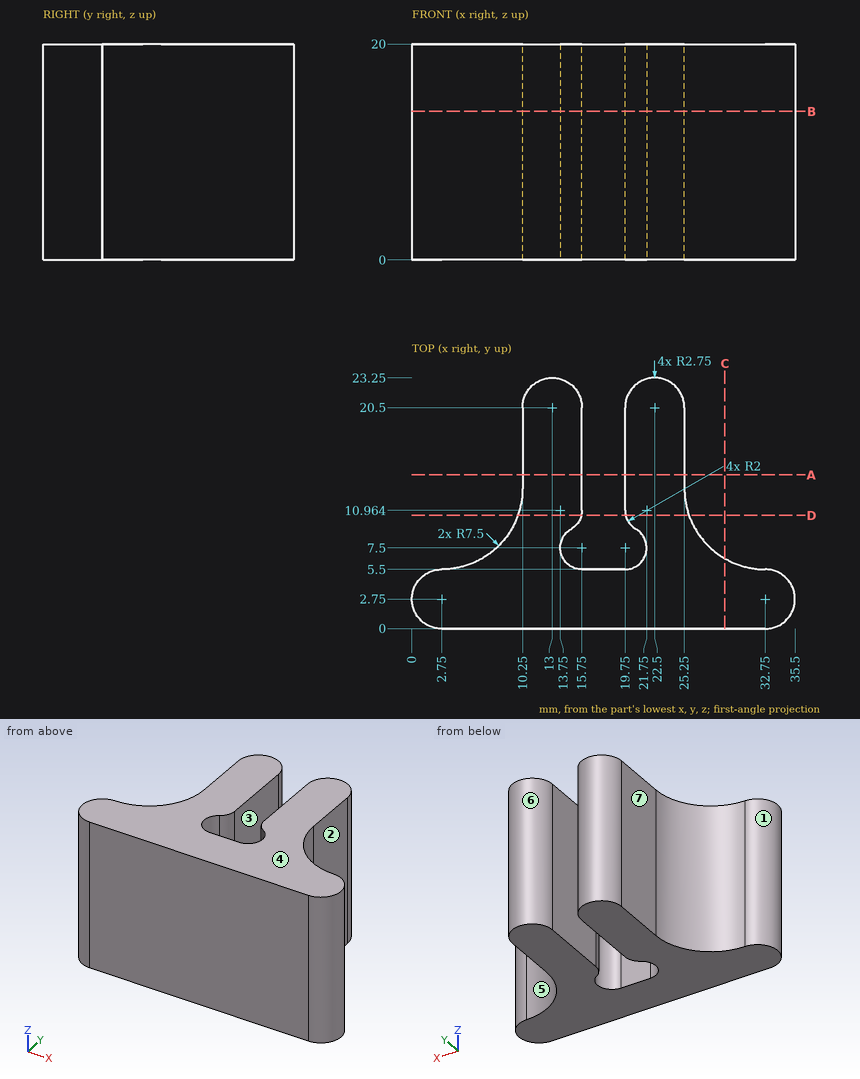
For this review, use the dimensioned drawing (mm, ordinates from the lowest corner) and the shaded views. A direction names the side the tool comes from. Give positions to 0.01 mm unless a question says otherwise; leave off trailing zeros. Order: outer loops, then holes, each group sorted by start corner. A loop starts at its lowest first (then second) coordinate and runs counter-clockwise, first axis right, second up. Notation, with made-up numbers: M 33,-40 L 85,-40 A12 ccw 85,-17 Z; hole C -22,62.5 d10. An arc over 180 degrees is marked long. Use one line per item in the form item = value. Start each with the question number.
Item 1: Insertion check: pin 1 Ø3 at (x, z) = (18, 15) entering from +Y; pin 2 Ø1 at (y, z) = (17, 8) entering from -X; pin 3 Ø1.5 at (y, z) = (15.5, 3.5) entering from +X. Each pin has a flat end and moves straight along its axis. Give the tip position at first contact, or say it passes through.
Item 2: We need section C-C on x = 29. Give the boundary of the cut face in (y, z) (3 decimals).
Item 3: For the marked faces 1, 2 and 3, list the 3-axis set-ups (+Z, -Z, +X, -X, +Y, -Y) from which the entire face can be reached by the end or side of a thin tool; tool diameter is ignored.
Item 4: We need section D-D on y = 10.5. Give the boundary of the cut face in (x, z), plus the area to 3 significant figures.
Item 5: The part is to be moulded in two halves that separate along X. For the marked faces 4, 5, 6 and 7, say which applies: pulls with the +X half, pulls with the -X half, needs draft (parallel to the pull), parting line crosses it, or undercut.
Item 6: To check wall thickness, follow line 1 along X through (y, z) = (15.5, 4); line 2 along X through (y, z) = (11.75, 1.5) (3 decimals); line 3 along Y through (x, z) = (21.5, 6). State the ranges of each line that lie inside material, in increasing order. Write a range as from..to.
Item 7: We need section A-A on y = 14.25. Give the boundary of the cut face in (x, z), plus the area to 3 significant figures.
Item 8: We need section B-B on z = 13.75. Give the boundary of the cut face in (x, y), plus the area to 3 significant figures.
Completed:
q1.pin_1 = 5.5
q1.pin_2 = 10.25
q1.pin_3 = 25.25
q2.outline = M 0,0 L 6.505,0 L 6.505,20 L 0,20 Z
q3.face_1 = +Z, -Z, -X
q3.face_2 = +Z, -Z, +X, +Y
q3.face_3 = +Z, -Z, +Y
q4.outline = M 9.82,0 L 15.7,0 L 15.7,20 L 9.82,20 Z; M 19.8,0 L 25.68,0 L 25.68,20 L 19.8,20 Z
q4.area = 235 mm²
q5.face_4 = needs draft
q5.face_5 = pulls with the +X half
q5.face_6 = undercut
q5.face_7 = pulls with the -X half
q6.line_1 = 10.25..15.75, 19.75..25.25
q6.line_2 = 10.145..15.75, 19.75..25.355
q6.line_3 = 0..6.53, 8.47..23.06
q7.outline = M 10.25,0 L 15.75,0 L 15.75,20 L 10.25,20 Z; M 19.75,0 L 25.25,0 L 25.25,20 L 19.75,20 Z
q7.area = 220 mm²
q8.outline = M 2.75,0 L 32.75,0 A2.75 ccw 32.75,5.5 A7.5 cw 25.25,13 L 25.25,20.5 A2.75 ccw 19.75,20.5 L 19.75,10.96 A2 ccw 20.75,9.23 A2 cw 19.75,5.5 L 15.75,5.5 A2 cw 14.75,9.23 A2 ccw 15.75,10.96 L 15.75,20.5 A2.75 ccw 10.25,20.5 L 10.25,13 A7.5 cw 2.75,5.5 A2.75 ccw Z
q8.area = 388 mm²
